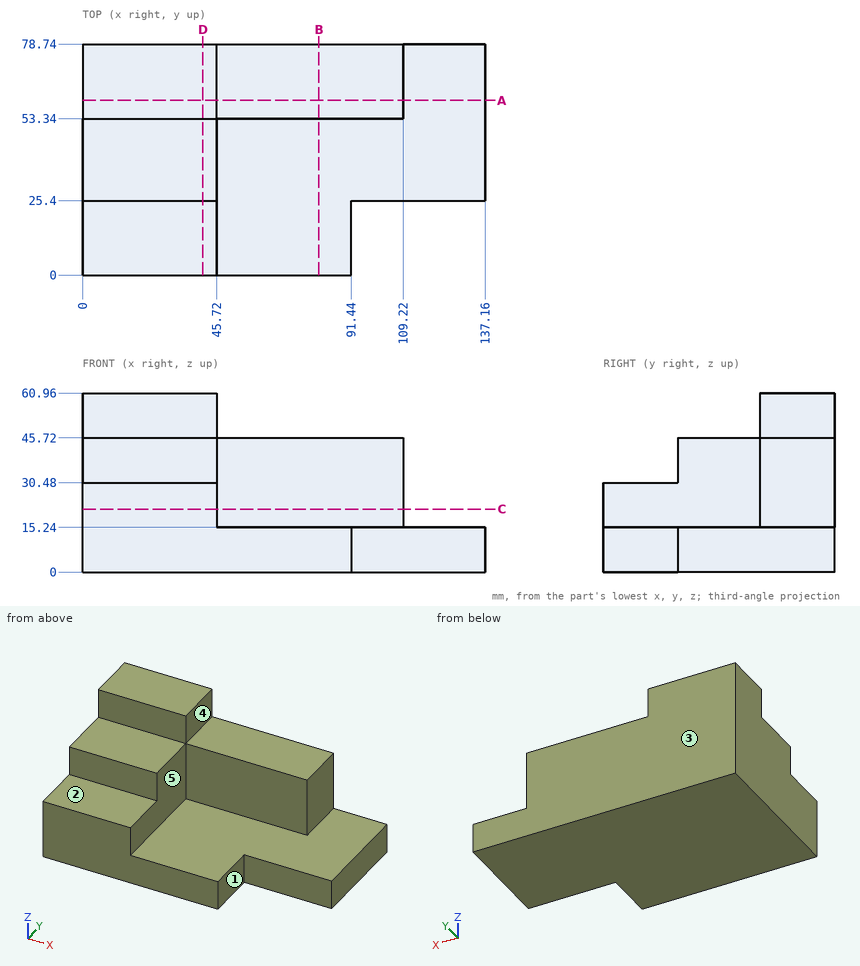
Design review of the part shown in the three views and the two pictorial views. Dimensions are in mm from the part's minimum x, y and z. A direction names the side the tool comes from. Round coordinates to 2 decimals unless told otherwise and drop trailing zeros. Write each loop counter-clockwise with the first axis right and the second up, starting at its lowest first coordinate (ties: lowest second). Pieces come first, ordered by that corner, then holes. Notation, with made-up numbers: M -14,7 L 9,7 A18 cw 9,41 Z; hole C 88,42 d8. An arc over 180 degrees is marked long. One line per item, written item: value. Start each with the question number.
1. Take a section at B-B on x = 80.5. State the section outline as (y, z) points, then the cut area to 3 significant figures.
2. Take a section at D-D on x = 41. State the section outline as (y, z) points, then the cut area to 3 significant figures.
3. Clearance check with flat-ended pins moving along their axes: P1, Ø7.5, axis at y = 10.5, z = 7.5, coming from the +X side; P2, Ø9, axis at y = 38, z = 26, coming from the +X side; P3, Ø7.5, axis at x = 78, y = 61, coming from the +Z side. State where each tip first meets the part, or that it passes through.
4. Take a section at C-C on z = 21.5. State the section outline as (x, y) points.
5. For the marked faces 1, 2, 3, 4 and 5, list the 3-axis set-ups (+Z, -Z, +X, -X, +Y, -Y) from which the entire face can be reached by the end or side of a thin tool; tool diameter is ignored.
6. Take a section at A-A on y = 59.5. State the section outline as (x, z) points, then the cut area to 3 significant figures.
7. To check wall thickness, follow probe 1 along Z at (x, y) = (66, 65); probe 2 along Z at (x, y) = (121, 27.5); probe 3 along X at (y, z) = (75, 17.5). State the ranges of each line that lie inside material, in increasing order. Write a range as from..to.
Computed:
1. outline: M 0,0 L 78.74,0 L 78.74,45.72 L 53.34,45.72 L 53.34,15.24 L 0,15.24 Z
1. area: 1,970 mm²
2. outline: M 0,0 L 78.74,0 L 78.74,60.96 L 53.34,60.96 L 53.34,45.72 L 25.4,45.72 L 25.4,30.48 L 0,30.48 Z
2. area: 3,600 mm²
3. P1: stops at x = 91.44
3. P2: stops at x = 45.72
3. P3: stops at z = 45.72
4. outline: M 0,0 L 45.72,0 L 45.72,53.34 L 109.22,53.34 L 109.22,78.74 L 0,78.74 Z
5. face 1: +Z, -Z, +X, -Y
5. face 2: +Z, +X, -X, -Y
5. face 3: +Z, -Z, +X, -X, +Y
5. face 4: +Z, +X, +Y, -Y
5. face 5: +Z, +X, -Y
6. outline: M 0,0 L 137.16,0 L 137.16,15.24 L 109.22,15.24 L 109.22,45.72 L 45.72,45.72 L 45.72,60.96 L 0,60.96 Z
6. area: 6,120 mm²
7. probe 1: z = 0..45.72
7. probe 2: z = 0..15.24
7. probe 3: x = 0..109.22
